Source: three-view drawing plus pictorial views. Frame: mm from the lowest corner of the part. A direction names the side the tool comes from. Coordinates: 2 decimals unless noted, no trailing zeros. Write each loop counter-clockwise with the first axis right and the second up, starting at its lowest first coordinate (ties: lowest second). Pieces come first, ordered by that corner, then holes. Notation, with made-up numbers: (-38.75, 79.25) -> (-23.75, 79.25) arc R16 cw to (-23.75, 85.25) -> close; hole circle Ø3 at (60.5, 59.25). An arc over 180 degrees is marked (long way). Write item = value, one per line.
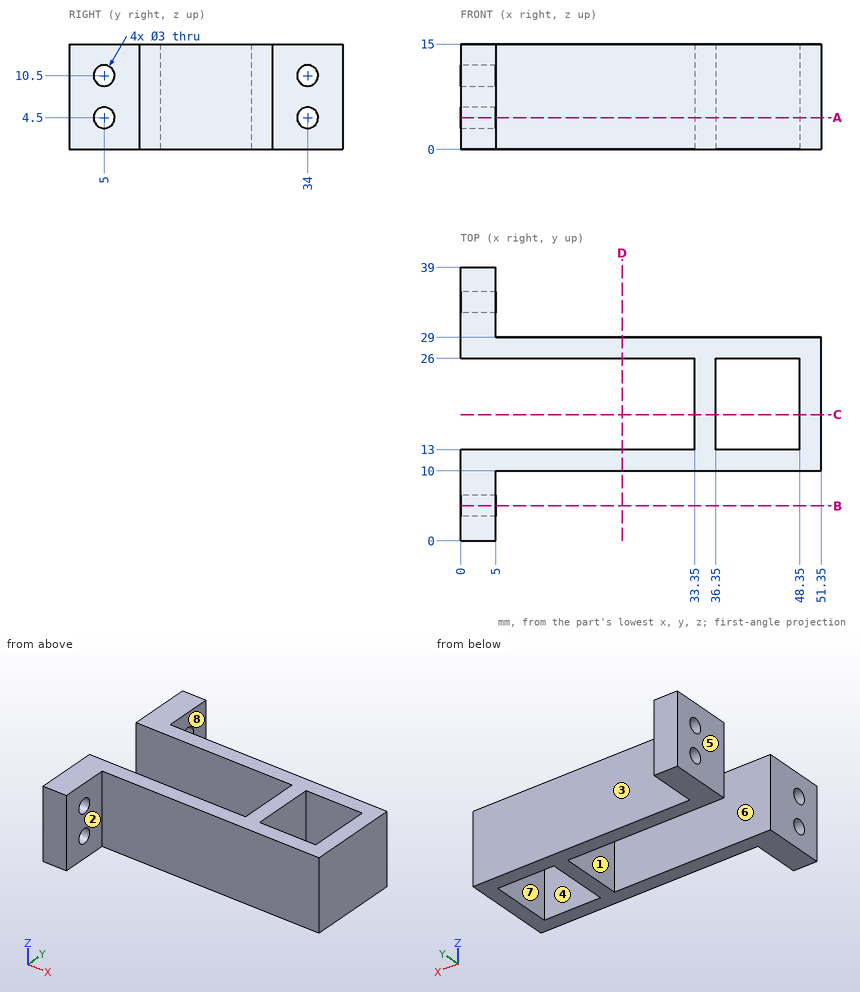
1) Cut plane C-C, the plane y = 18. Output: boundary loops of the cut face in (x, z).
Answer block:
outline = (33.35, 0) -> (36.35, 0) -> (36.35, 15) -> (33.35, 15) -> close; (48.35, 0) -> (51.35, 0) -> (51.35, 15) -> (48.35, 15) -> close
2) Cut plane A-A, the plane z = 4.5. Output: boundary loops of the cut face in (x, y), and give its area (3 significant figures).
Answer block:
outline = (0, 0) -> (5, 0) -> (5, 3.5) -> (0, 3.5) -> close; (0, 6.5) -> (5, 6.5) -> (5, 10) -> (51.35, 10) -> (51.35, 29) -> (5, 29) -> (5, 32.5) -> (0, 32.5) -> (0, 26) -> (33.35, 26) -> (33.35, 13) -> (0, 13) -> close; (0, 35.5) -> (5, 35.5) -> (5, 39) -> (0, 39) -> close; hole (36.35, 13) -> (48.35, 13) -> (48.35, 26) -> (36.35, 26) -> close
area = 456 mm2
3) Material intervals for probe 1 along Y at (x, z) = (1.65, 4.5); probe 2 along X at (y, z) = (15, 6.25); probe 3 along Y at (x, z) = (29, 4.75), sorted ascending. Write a range as [from, to].
Answer block:
probe_1 = [0, 3.5], [6.5, 13], [26, 32.5], [35.5, 39]
probe_2 = [33.35, 36.35], [48.35, 51.35]
probe_3 = [10, 13], [26, 29]
4) Cut plane D-D, the plane x = 23. Output: boundary loops of the cut face in (y, z), and give its area (3 significant figures).
Answer block:
outline = (10, 0) -> (13, 0) -> (13, 15) -> (10, 15) -> close; (26, 0) -> (29, 0) -> (29, 15) -> (26, 15) -> close
area = 90.0 mm2
5) Pull-direction query (X, two-part tool) for the marked faces 5, 6, 7 and 8; classes: +X half, -X half, draft (parallel to the pull), parting line (faces both ways), or undercut.
Answer block:
face_5 = -X half
face_6 = draft
face_7 = undercut
face_8 = +X half
6) First-contact query: pin 1 Ø6 at (x, z) = (6, 8.5) entering from +Y; pin 2 Ø5 at (x, z) = (45, 8.5) entering from -Y; pin 3 Ø8 at (y, z) = (36, 6.5) entering from +X; pin 4 Ø2.5 at (y, z) = (5, 10.5) entering from -X. Flat tips, straight axial feed; report the tip coordinate or a pass-through.
Answer block:
pin_1 = 39
pin_2 = 10
pin_3 = 5
pin_4 = through
7) Cut plane B-B, the plane y = 5. Output: boundary loops of the cut face in (x, z), and give its area (3 significant figures).
Answer block:
outline = (0, 0) -> (5, 0) -> (5, 3) -> (0, 3) -> close; (0, 6) -> (5, 6) -> (5, 9) -> (0, 9) -> close; (0, 12) -> (5, 12) -> (5, 15) -> (0, 15) -> close
area = 45.0 mm2
8) Reachability of the marked faces 1, 2, 3 and 4 from +Z, -Z, +X, -X, +Y, -Y: full face, straight path, thin tool, end or side. Return the list, or none.
Answer block:
face_1 = +Z, -Z, -X
face_2 = +Z, -Z, +X, -Y
face_3 = +Z, -Z, +X, +Y
face_4 = +Z, -Z
